```python
from build123d import *

# Parameters (mm, degrees)
CROQUIS1_R              = 1.585
CROQUIS1_R_2            = 1.5
SALIENTE_EXTRUIR1_DEPTH = 5
CROQUIS2_R              = 1.5
CORTAR_EXTRUIR1_DEPTH   = 35


with BuildPart() as part:
    # Croquis1 → Saliente-Extruir1 (new body)
    with BuildSketch(Plane.XY):
        with BuildLine():
            Line((-13.632801604, 23.936623068), (-13.632801604, 2.936623068))
            Line((-13.632801604, 2.936623068), (-13.632801604, -7.763376932))
            Line((-13.632801604, -7.763376932), (13.717198396, -7.763376932))
            ThreePointArc((13.717198396, -7.763376932), (17.54403272, -7.002172257), (20.788266208, -4.834444744))
            Line((20.788266208, -4.834444744), (20.788266208, 21.00769088))
            ThreePointArc((20.788266208, 21.00769088), (17.54403272, 23.175418393), (13.717198396, 23.936623068))
            Line((13.717198396, 23.936623068), (-13.632801604, 23.936623068))
        make_face()
        with Locations((7.867198396, 8.086623068)):
            Circle(CROQUIS1_R, mode=Mode.SUBTRACT)
        with Locations((-0.132801604, 8.086623068)):
            Circle(CROQUIS1_R_2, mode=Mode.SUBTRACT)
        with Locations((7.867198396, -1.413376932)):
            Circle(CROQUIS1_R_2, mode=Mode.SUBTRACT)
        with Locations((15.867198396, 8.086623068)):
            Circle(CROQUIS1_R_2, mode=Mode.SUBTRACT)
        with Locations((7.867198396, 17.586623068)):
            Circle(CROQUIS1_R_2, mode=Mode.SUBTRACT)
        with Locations((-9.132801604, 7.236623068)):
            Circle(CROQUIS1_R_2, mode=Mode.SUBTRACT)
        with Locations((-9.132801604, -2.763376932)):
            Circle(CROQUIS1_R_2, mode=Mode.SUBTRACT)
    extrude(amount=SALIENTE_EXTRUIR1_DEPTH)

    # Croquis2 → Cortar-Extruir1 (cut)
    with BuildSketch(Plane(origin=(0, 23.936623068, 0), x_dir=(1, 0, 0), z_dir=(0, 1, 0))):
        with Locations(Location((7.867198396, -2.682084827, 0), (0, 0, 270))):
            Circle(CROQUIS2_R)
    extrude(amount=-CORTAR_EXTRUIR1_DEPTH, mode=Mode.SUBTRACT)


solid = part.part
```
Verification items for the finished model (mm, model axes). Coordinates: 2 decimals unless noted, no trailing zeros. Order: outer loops, then holes, each group sorted by start corner. A loop starts at its lowest first (then second) coordinate and runs counter-clockwise, first axis right, second up. Notation, with made-up numbers: (-6.5, -13.75) -> (42.5, -13.75) arc R19 ccw to (42.5, 1.25) -> close; hole circle Ø9 at (16, 87). An arc over 180 degrees is marked (long way). Put each result on its own line as item: value. Start each with the question number.
1) Cross-section at C-C (x = 7). State how many separate pieces and enclosed holes the cut face has, plus the area to 3 significant figures.
2) Cross-section at D-D (y = 5). Enter the section's corners in (x, z).
3) Cross-section at A-A (z = 2.1). Enter the section's corners in (x, y) (3 decimals).
4) Release check for a two-part mould opening along Z. For faces 1 (the cylindrical face through (9.13, -5.25, 3.49)), 2 (the cylindrical face through (7.293, 13.156, 4.068)), 3 (the flat face through (3, 8, 0)), 4 (the flat face through (20.788, 8, 2)) record: pulls with the +Z half, pulls with the -Z half, needs draft (parallel to the pull), parting line crosses it, or undercut.
5) Material ranges on L1, parallel to Y at x = -9, z = 1.95; L2, parallel to Y at x = -10.5, z = 0.8; L3, parallel to X at y = 7, z = 2.55, recorded low to high.
6) Cross-section at B-B (y = 17). Enter the section's corners in (x, z), plus the area to 3 significant figures.
Geometry check:
1. separate pieces: 8
1. enclosed holes: 0
1. area: 61.6 mm^2
2. outline: (-13.63, 0) -> (20.79, 0) -> (20.79, 5) -> (-13.63, 5) -> close; hole circle Ø3 at (7.87, 2.68)
3. outline: (-13.633, -7.763) -> (6.485, -7.763) -> (6.485, -1.995) arc R1.5 cw to (6.485, -0.831) -> (6.485, 7.311) arc R1.585 cw to (6.485, 8.862) -> (6.485, 17.005) arc R1.5 cw to (6.485, 18.169) -> (6.485, 23.937) -> (-13.633, 23.937) -> close; (9.25, -7.763) -> (13.717, -7.763) arc R10 ccw to (20.788, -4.834) -> (20.788, 21.008) arc R10 ccw to (13.717, 23.937) -> (9.25, 23.937) -> (9.25, 18.169) arc R1.5 cw to (9.25, 17.005) -> (9.25, 8.862) arc R1.585 cw to (9.25, 7.311) -> (9.25, -0.831) arc R1.5 cw to (9.25, -1.995) -> close; hole circle Ø3 at (-9.133, -2.763); hole circle Ø3 at (-9.133, 7.237); hole circle Ø3 at (-0.133, 8.087); hole circle Ø3 at (15.867, 8.087)
4. face 1: undercut
4. face 2: undercut
4. face 3: pulls with the -Z half
4. face 4: needs draft
5. L1: y = -7.76 to -4.26, -1.27 to 5.74, 8.73 to 23.94
5. L2: y = -7.76 to -3.38, -2.15 to 6.62, 7.85 to 23.94
5. L3: x = -13.63 to -10.61, -7.65 to -1.17, 0.9 to 6.37, 9.36 to 14.83, 16.9 to 20.79
6. outline: (-13.63, 0) -> (6.49, 0) -> (6.49, 2.1) arc R1.5 cw to (6.49, 3.27) -> (6.49, 5) -> (-13.63, 5) -> close; (9.25, 0) -> (20.79, 0) -> (20.79, 5) -> (9.25, 5) -> (9.25, 3.27) arc R1.5 cw to (9.25, 2.1) -> close
6. area: 158 mm^2
